CAD build for the part. Positions are in the model's coordinates, mm. Coordinates: 2 decimals unless noted, no trailing zeros. Write each loop counter-clockwise with the first axis right and the second up, starting at its lowest first coordinate (ties: lowest second). Pieces come first, ordered by that corner, then holes. Notation, with made-up numbers: (65, 84) - (84, 84) arc R14 cw to (84, 95) - close; hole circle Ø4 at (68.25, -9.75). An arc over 180 degrees is marked (long way). Answer in a Markdown table with one row per item. Add a question column.
Q1. Band-saw the part on A-A (z = -50.8). List the corners of the cut face in (x, y) (3 decimals), and give its area (3 significant figures).
Q2. Pin check, flat tip, straight feed: pin 1 (6.5 mm diameter, centred on x = -66.04, z = -50.8, fed in from +Y) (3 decimals). Stop position of the tip, or through.
Q3. Drill centre lines: line 1 along Z through (x, y) = (-66.04, 0.8) (3 decimals); line 2 along Z through (x, y) = (-33.02, 2) (3 decimals); line 3 along X through (y, z) = (1.1, -35). Where is each one in solid material? Low to high. Write a range as from..to.
Q4. Two-plate mould, pull along X, no slides. Class faces 1 (the cylindrical face through (-34.946, 1.565, -11.719)), 2 (the cylindrical face through (-7.18, 1.57, -34.54)), 3 (the flat face through (-39, 0, -23)), 4 (the flat face through (-78.74, 2, -23)): +X half, -X half, draft (parallel to the pull), parting line (faces both ways), or undercut.
Q5. Band-saw the part on B-B (x = -33.02). List the corners of the cut face in (y, z) (3 decimals), and give its area (3 significant figures).
Q6. Band-saw the part on D-D (x = -66.04). List the corners of the cut face in (y, z) (3 decimals).
Q7. Band-saw the part on C-C (y = 1.1). List the corners of the cut face in (x, z) (1 decimal).
Autodesk Inventor part; units mm, degrees
ref_plane "YZ Plane" through (0, 0, 0) normal (1, 0, 0) x (0, 1, 0)
ref_plane "XZ Plane" through (0, 0, 0) normal (0, 1, 0) x (-1, 0, 0)
ref_plane "XY Plane" through (0, 0, 0) normal (0, 0, 1) x (1, 0, 0)
sketch "Sketch1" plane through (0, 0, 0) normal (0, 1, 0) x (-1, 0, 0)
  line L0 (0, 0) -> (101.6, 0)
  line L1 (101.6, 0) -> (101.6, -47.625)
  line L2 (101.6, -47.625) -> (0, -47.625)
  line L3 (0, -47.625) -> (0, 0)
  circle A0 centre (88.9, -9.525) radius 2.5
  circle A1 centre (88.9, -38.1) radius 2.5
  circle A2 centre (7.62, -11.1125) radius 2.0193
  circle A3 centre (33.02, -11.1125) radius 2.0193
  circle A4 centre (33.02, -36.5125) radius 2.0193
  circle A5 centre (7.62, -36.5125) radius 2.0193
  line L4 (0, 0) -> (0, -40.7836)
  point P0 (37.1991, -51.2989)
  point P1 (24.9809, -31.7225)
  point P2 (38.4109, -31.7225)
  dimension "d0" = 101.6
  dimension "d1" = 47.625
  dimension "d2" = 5
  dimension "d3" = 5
  dimension "d4" = 12.7
  dimension "d5" = 12.7
  dimension "d6" = 9.525
  dimension "d7" = 9.525
  dimension "d8" = 25.4
  dimension "d9" = 25.4
  dimension "d10" = 25.4
  dimension "d11" = 25.4
  dimension "d12" = 4.0386
  dimension "d13" = 4.0386
  dimension "d14" = 4.0386
  dimension "d15" = 4.0386
  dimension "d16" = 11.1125
extrude "Extrusion1" add sketch "Sketch1" along normal blind 3.175
sketch "Sketch2" plane through (0, 3.175, 0) normal (0, 1, 0) x (1, 0, 0)
  line L0 (-101.6, 47.625) -> (-101.6, 0)
  line L1 (-101.6, 0) -> (0, 0)
  line L2 (0, 0) -> (0, 47.625)
  line L3 (0, 47.625) -> (-101.6, 47.625)
  circle A0 centre (-88.9, 9.525) radius 2.5
  circle A1 centre (-88.9, 38.1) radius 2.5
  circle A2 centre (-7.62, 11.1125) radius 2.0193
  circle A3 centre (-33.02, 11.1125) radius 2.0193
  circle A4 centre (-33.02, 36.5125) radius 2.0193
  circle A5 centre (-7.62, 36.5125) radius 2.0193
  line L4 (-78.74, 0) -> (-78.74, 47.625)
  line L5 (0, 47.625) -> (-101.6, 47.625)
  line L6 (0, -12.7) -> (-78.74, -12.7)
  line L7 (-78.74, -12.7) -> (-78.74, 60.325)
  line L8 (-78.74, 60.325) -> (0, 60.325)
  line L9 (0, 60.325) -> (0, -12.7)
  circle A6 centre (-66.04, -3.175) radius 2.5
  circle A7 centre (-66.04, 50.8) radius 2.5
  dimension "d19" = 78.74
  dimension "d20" = 9.525
  dimension "d21" = 12.7
  dimension "d22" = 12.7
  dimension "d23" = 9.525
  dimension "d24" = 12.7
  dimension "d25" = 12.7
extrude "Extrusion2" add sketch "Sketch2" against normal blind 3.175 contours L7 L8 L9 L3 | L3 L2 L1 L4 | L1 L9 L6 L7
extrude "Extrusion3" cut sketch "Sketch2" against normal through all contours L3 L4 L1 L0
equation "\"d5\" = d4"
equation "\"d6\" = 0.2 * d1"
equation "\"d7\" = d6"
equation "\"d20\" = d7"
equation "\"d21\" = d5"
equation "\"d23\" = d20"
equation "\"d25\" = d24"
properties part number "MotorMount" material "Aluminum 6061"
Checked values:
| question | item | result |
|---|---|---|
| 1 | outline | (-78.74, 0) - (-68.54, 0) - (-68.54, 3.175) - (-78.74, 3.175) - close; (-63.54, 0) - (0, 0) - (0, 3.175) - (-63.54, 3.175) - close |
| 1 | area | 234 mm² |
| 2 | pin 1 | stops at y = 3.175 |
| 3 | line 1 | z = -60.325..-53.3, -48.3..0.675, 5.675..12.7 |
| 3 | line 2 | z = -60.325..-38.532, -34.493..-13.132, -9.093..12.7 |
| 3 | line 3 | x = -78.74..-34.36, -31.68..-8.96, -6.28..0 |
| 4 | face 1 | undercut |
| 4 | face 2 | undercut |
| 4 | face 3 | draft |
| 4 | face 4 | -X half |
| 5 | outline | (0, -60.325) - (3.175, -60.325) - (3.175, -38.532) - (0, -38.532) - close; (0, -34.493) - (3.175, -34.493) - (3.175, -13.132) - (0, -13.132) - close; (0, -9.093) - (3.175, -9.093) - (3.175, 12.7) - (0, 12.7) - close |
| 5 | area | 206 mm² |
| 6 | outline | (0, -60.325) - (3.175, -60.325) - (3.175, -53.3) - (0, -53.3) - close; (0, -48.3) - (3.175, -48.3) - (3.175, 0.675) - (0, 0.675) - close; (0, 5.675) - (3.175, 5.675) - (3.175, 12.7) - (0, 12.7) - close |
| 7 | outline | (-78.7, -60.3) - (0, -60.3) - (0, 12.7) - (-78.7, 12.7) - close; hole circle Ø5 at (-66, -50.8); hole circle Ø5 at (-66, 3.2); hole circle Ø4 at (-33, -36.5); hole circle Ø4 at (-33, -11.1); hole circle Ø4 at (-7.6, -36.5); hole circle Ø4 at (-7.6, -11.1) |
